Autodesk Fusion 360 part; units mm, degrees
sketch "Sketch1" plane through (0, 0, 0) normal (0, 0, 1) x (1, 0, 0)
  line L0 (22.28, -10.39) -> (-22.28, -10.39) construction
  line L1 (-22.28, -10.39) -> (-22.28, 10.39) construction
  line L2 (-22.28, 10.39) -> (22.28, 10.39) construction
  line L3 (22.28, 10.39) -> (22.28, -10.39) construction
  line L4 (22.28, -10.39) -> (-22.28, 10.39) construction
  line L5 (-22.28, -10.39) -> (22.28, 10.39) construction
  circle A0 centre (22.28, 10.39) radius 5
  circle A1 centre (22.28, -10.39) radius 5
  circle A2 centre (-22.28, -10.39) radius 5
  circle A3 centre (-22.28, 10.39) radius 5
  line L6 (-22.28, 15.39) -> (22.28, 15.39)
  line L7 (-27.28, 10.39) -> (-27.28, -10.39)
  line L8 (27.28, 10.39) -> (27.28, -10.39)
  line L9 (-22.28, -15.39) -> (22.28, -15.39)
  circle A4 centre (22.28, 10.39) radius 2.7
  circle A5 centre (-22.28, 10.39) radius 2.7
  circle A6 centre (-22.28, -10.39) radius 2.7
  circle A7 centre (22.28, -10.39) radius 2.7
  dimension "d1" = 44.56
  dimension "d2" = 20.78
  dimension "d3" = 10
  dimension "d4" = 10
  dimension "d5" = 10
  dimension "d6" = 10
  dimension "d12" = 5.4
  dimension "d13" = 5.4
  dimension "d14" = 5.4
  dimension "d15" = 5.4
extrude "Extrude1" add sketch "Sketch1" along normal blind 3 contours A0 | A0 A1 A2 A3 L6 L7 L8 L9 | A1 | A3 | A2 | A4 | A5 | A6 | A7
extrude "Extrude2" add sketch "Sketch1" along normal blind 6 from surface at 3 contours A0 | A1 | A3 | A2 | A4 | A5 | A6 | A7
extrude "Extrude3" cut sketch "Sketch1" against normal blind 7 from surface at 9 contours A4 | A5 | A6 | A7
equation "d4 = d3"
equation "d5 = d3"
equation "d6 = d3"
equation "d13 = d12"
equation "d14 = d12"
equation "d15 = d12"
Read the model definition and answer for the solid it produces. Units are mm, in the model's axes. A direction names the side the tool comes from. Round coordinates to 2 decimals unless told otherwise and drop trailing zeros. Write each loop counter-clockwise with the first axis right and the second up, starting at its lowest first coordinate (ties: lowest second). Pieces come first, ordered by that corner, then holes. Notation, with made-up numbers: M 60.5,-30 L 64.5,-30 A33 ccw 64.5,8 Z; hole C 18.25,-20.75 d4. An arc over 180 degrees is marked long. One line per item, written item: value.
Q1. For a pull along X with two mould halves and no side action, classify faces 3 (the flat face through (-20, 8, 9)), 4 (the flat face through (27.28, 0, 1)), 5 (the flat face through (-22, 10, 2)) as +X half, -X half, draft (parallel to the pull), parting line (faces both ways), or undercut.
Data:
face 3: draft
face 4: +X half
face 5: undercut
Q2. Straight lines are drawn through the part: line 1 (Y direction, x = -22.28, z = 5); line 2 (X direction, y = -10.5, z = 3.75); line 3 (X direction, y = 10, z = 2.5). For each, find the intervals that lie inside material, in ascending order. Write a range as [from, to].
Data:
line 1: [-15.39, -13.09], [-7.69, -5.39], [5.39, 7.69], [13.09, 15.39]
line 2: [-27.28, -24.98], [-19.58, -17.28], [17.28, 19.58], [24.98, 27.28]
line 3: [-27.28, -24.95], [-19.61, 19.61], [24.95, 27.28]
Q3. Find section D-D on y = 0. Write down the section's boundary in (x, z).
Data:
outline: M -27.28,0 L 27.28,0 L 27.28,3 L -27.28,3 Z
Q4. Find section B-B on x = -21.5. Write down the section's boundary in (y, z).
Data:
outline: M -15.39,0 L 15.39,0 L 15.39,3 L 15.33,3 L 15.33,9 L 12.97,9 L 12.97,2 L 7.81,2 L 7.81,9 L 5.45,9 L 5.45,3 L -5.45,3 L -5.45,9 L -7.81,9 L -7.81,2 L -12.97,2 L -12.97,9 L -15.33,9 L -15.33,3 L -15.39,3 Z
Q5. Which of the six approach directions +Z, -Z, +X, -X, +Y, -Y give full straight-line access (tool end or side, diameter ignored) to faces 1 (the cylindrical face through (26.9, 12.3, 5.4)), 2 (the flat face through (-27.28, 0, 1))?
Data:
face 1: +Z
face 2: +Z, -Z, -X, +Y, -Y
Q6. Flat-ended cylindrical pins translate along their axes: pin 1 Ø2.5 at (x, y) = (-22, -10) entering from +Z; pin 2 Ø4 at (x, y) = (2.5, 5.5) entering from +Z. Find the tip coordinate at first contact, or state that the pin passes through.
Data:
pin 1: z = 2
pin 2: z = 3
Q7. Find section A-A on z = 4.5. Write down the section's boundary in (x, y).
Data:
outline: C -22.28,-10.39 d10; C -22.28,10.39 d10; C 22.28,-10.39 d10; C 22.28,10.39 d10; hole C -22.28,-10.39 d5.4; hole C -22.28,10.39 d5.4; hole C 22.28,-10.39 d5.4; hole C 22.28,10.39 d5.4
Q8. Find section C-C on y = 11.5. Write down the section's boundary in (x, z), plus the area to 3 significant figures.
Data:
outline: M -27.16,0 L 27.16,0 L 27.16,9 L 24.74,9 L 24.74,2 L 19.82,2 L 19.82,9 L 17.4,9 L 17.4,3 L -17.4,3 L -17.4,9 L -19.82,9 L -19.82,2 L -24.74,2 L -24.74,9 L -27.16,9 Z
area: 211 mm2
